Build history of the part. All positions in model axes, mm. Round coordinates to 2 decimals unless told otherwise and drop trailing zeros. Order: outer loops, then holes, each group sorted by start corner. A loop starts at its lowest first (then second) coordinate and runs counter-clockwise, first axis right, second up. Notation, with made-up numbers: (2.5, 85) -> (47.5, 85) arc R22 ccw to (47.5, 123) -> close; hole circle Ø8 at (34.25, -37). An arc over 180 degrees is marked (long way). Answer as a JSON object with one key per item and string values.
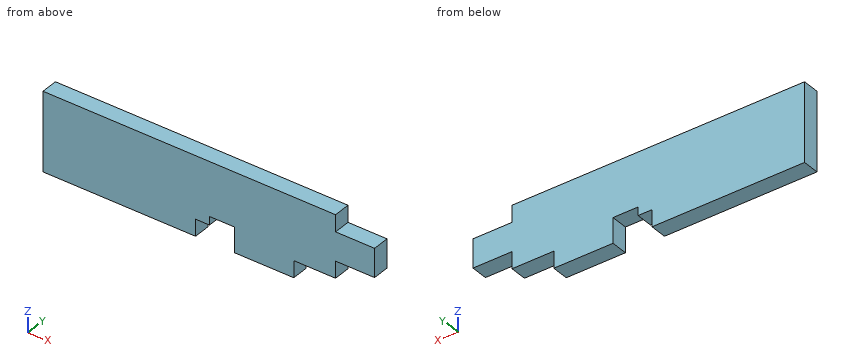
from build123d import *

# Parameters (mm, degrees)
SKETCH1_W           = 666.75
SKETCH1_H           = 179.3875
BOSS_EXTRUDE1_DEPTH = 38.1
SKETCH2_W           = 88.9
SKETCH2_H           = 141.2875
BOSS_EXTRUDE2_DEPTH = 38.1
SKETCH3_W           = 184.15
SKETCH3_H           = 38.1
CUT_EXTRUDE1_DEPTH  = 39.1
CUT_EXTRUDE2_DEPTH  = 39.1
SKETCH5_W           = 88.9
SKETCH5_H           = 38.1
CUT_EXTRUDE3_DEPTH  = 39.1


with BuildPart() as part:
    # Sketch1 → Boss-Extrude1 (new body)
    with BuildSketch(Plane(origin=(0, 0, 0), x_dir=(1, 0, 0), z_dir=(0, 1, 0))):
        with Locations((333.375, 89.69375)):
            Rectangle(SKETCH1_W, SKETCH1_H)
    extrude(amount=BOSS_EXTRUDE1_DEPTH)

    # Sketch2 → Boss-Extrude2 (add, through all)
    with BuildSketch(Plane.XZ):
        with Locations((711.2, -108.74375)):
            Rectangle(SKETCH2_W, SKETCH2_H)
    extrude(amount=-BOSS_EXTRUDE2_DEPTH)

    # Sketch3 → Cut-Extrude1 (cut, through all)
    with BuildSketch(Plane.XZ):
        with Locations((663.575, -160.3375)):
            Rectangle(SKETCH3_W, SKETCH3_H)
    extrude(amount=-CUT_EXTRUDE1_DEPTH, mode=Mode.SUBTRACT)

    # Sketch4 → Cut-Extrude2 (cut, through all)
    with BuildSketch(Plane.XZ):
        Polygon((436.55104079, -141.2875), (436.55104079, -122.2375), (379.4125, -122.2375), (379.4125, -141.2875), (347.6625, -141.2875), (347.6625, -179.3875), (436.55104079, -179.3875), align=None)
    extrude(amount=-CUT_EXTRUDE2_DEPTH, mode=Mode.SUBTRACT)

    # Sketch5 → Cut-Extrude3 (cut, through all)
    with BuildSketch(Plane.XZ):
        with Locations((711.2, -122.2375)):
            Rectangle(SKETCH5_W, SKETCH5_H)
    extrude(amount=-CUT_EXTRUDE3_DEPTH, mode=Mode.SUBTRACT)


solid = part.part
1) Flat gauge pins, fed straight in: pin 1 Ø16 at (x, y) = (361.5, 28) entering from -Z; pin 2 Ø11.5 at (y, z) = (16.5, -168.5) entering from +X; pin 3 Ø5.5 at (y, z) = (10.5, -134.5) entering from +X. Where does each tip first touch, or does it go through?
Checked values:
{"pin 1": "stops at z = -141.29", "pin 2": "stops at x = 571.5", "pin 3": "stops at x = 666.75"}
2) Probe L1, parallel to X at y = 15.5, z = -133.5; L2, parallel to X at y = 16.5, z = -144; L3, parallel to X at y = 11, z = -103.5. List the from-to ranges inside material, lowest first. Write a range as from..to.
Checked values:
{"L1": "x = 0..379.41, 436.55..666.75", "L2": "x = 0..347.66, 436.55..571.5", "L3": "x = 0..666.75"}
3) Cut at A-A, the plane z = -159.5. Give the cut face in (x, y), plus the area to 3 significant figures.
Checked values:
{"outline": "(0, 0) -> (347.66, 0) -> (347.66, 38.1) -> (0, 38.1) -> close; (436.55, 0) -> (571.5, 0) -> (571.5, 38.1) -> (436.55, 38.1) -> close", "area": "18,400 mm²"}
4) Cut at B-B, the plane y = 13.5. Give the cut face in (x, z).
Checked values:
{"outline": "(0, -179.39) -> (347.66, -179.39) -> (347.66, -141.29) -> (379.41, -141.29) -> (379.41, -122.24) -> (436.55, -122.24) -> (436.55, -179.39) -> (571.5, -179.39) -> (571.5, -141.29) -> (666.75, -141.29) -> (666.75, -103.19) -> (755.65, -103.19) -> (755.65, -38.1) -> (666.75, -38.1) -> (666.75, 0) -> (0, 0) -> close"}
5) Cut at C-C, the plane x = 688. Give the cut face in (y, z), plus the area to 3 significant figures.
Checked values:
{"outline": "(0, -103.19) -> (38.1, -103.19) -> (38.1, -38.1) -> (0, -38.1) -> close", "area": "2,480 mm²"}
